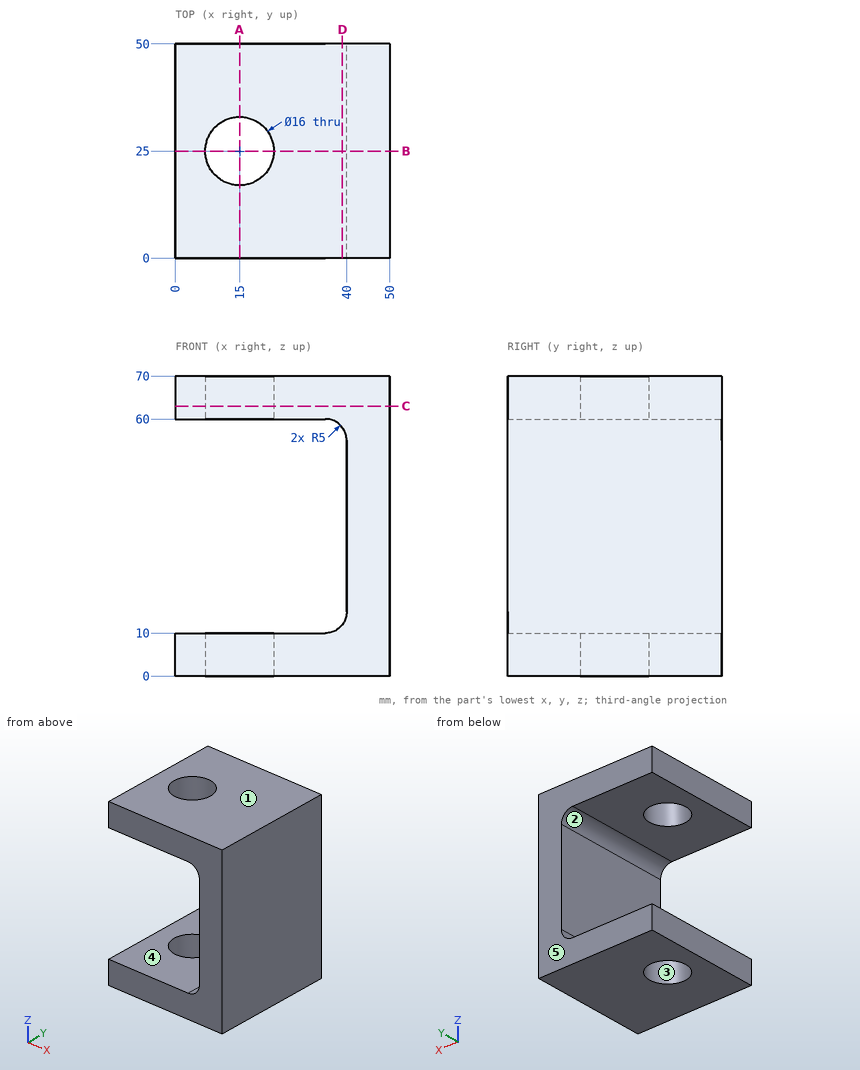
Here's the drawing with two shaded views (mm, measured from the low corner). I have some questions. A direction names the side the tool comes from. Give positions to 0.01 mm unless a question says otherwise; leave off trailing zeros. Loops run counter-clockwise (first coordinate to the right, second up) from the corner with the lowest first, then second, coordinate; pieces in that order, holes last. Notation, with made-up numbers: (74, 17) - (113, 17) arc R8 cw to (113, 31) - close; hole circle Ø9 at (39.5, 89). An arc over 180 degrees is marked (long way). Return JSON: item names as keys, results as strings.
1. I want a section at B-B on y = 25. Please give me the cut outline in (x, z), and give its area (3 significant figures).
Output values:
{"outline": "(0, 0) - (7, 0) - (7, 10) - (0, 10) - close; (0, 60) - (7, 60) - (7, 70) - (0, 70) - close; (23, 0) - (50, 0) - (50, 70) - (23, 70) - (23, 60) - (35, 60) arc R5 cw to (40, 55) - (40, 15) arc R5 cw to (35, 10) - (23, 10) - close", "area": "1,190 mm²"}
2. We'd pull the mould along Y, two halves only. Please class the marked faces 3, 4 and 5: +Y half, -Y half, draft (parallel to the pull), parting line (faces both ways), or undercut.
Output values:
{"face 3": "undercut", "face 4": "draft", "face 5": "+Y half"}
3. I want a section at D-D on x = 39. Please give me the cut outline in (y, z), and give its area (3 significant figures).
Output values:
{"outline": "(0, 0) - (50, 0) - (50, 12) - (0, 12) - close; (0, 58) - (50, 58) - (50, 70) - (0, 70) - close", "area": "1,200 mm²"}
4. I want a section at A-A on x = 15. Please give me the cut outline in (y, z).
Output values:
{"outline": "(0, 0) - (17, 0) - (17, 10) - (0, 10) - close; (0, 60) - (17, 60) - (17, 70) - (0, 70) - close; (33, 0) - (50, 0) - (50, 10) - (33, 10) - close; (33, 60) - (50, 60) - (50, 70) - (33, 70) - close"}
5. If I drill on line 1 (Z direction, x = 4.5, y = 41.5); line 2 (Y direction, x = 15, z = 7.75); line 3 (X direction, y = 11.5, z = 53.5), over which ranges is the centre line in solid material (lowest first)?
Output values:
{"line 1": "z = 0 to 10, 60 to 70", "line 2": "y = 0 to 17, 33 to 50", "line 3": "x = 40 to 50"}
6. I want a section at C-C on z = 63. Please give me the cut outline in (x, y), and give its area (3 significant figures).
Output values:
{"outline": "(0, 0) - (50, 0) - (50, 50) - (0, 50) - close; hole circle Ø16 at (15, 25)", "area": "2,300 mm²"}
7. I'm going to push a flat-ended pin straight in: pin 1 Ø8 at (y, z) = (12.5, 45) entering from -X. Where does the tip first touch, or does it pass through?
Output values:
{"pin 1": "stops at x = 40"}
8. For the marked faces 1 and 2, which set-ups out of +Z, -Z, +X, -X, +Y, -Y let a thin tool reach every point of the face, with its end or its side?
Output values:
{"face 1": "+Z, +X, -X, +Y, -Y", "face 2": "-X, +Y, -Y"}
